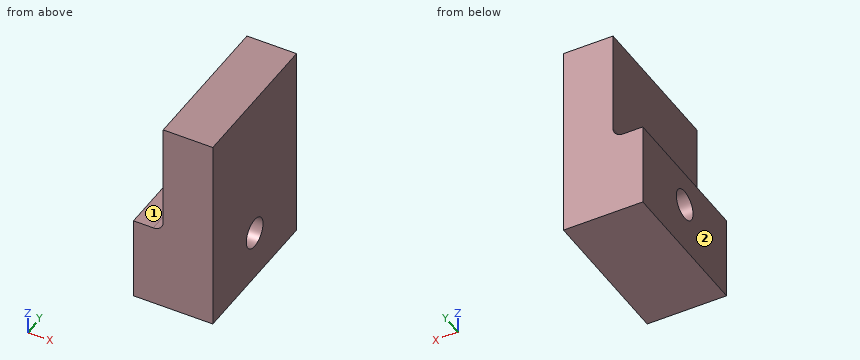
```python
from build123d import *

# Parameters (mm, degrees)
EXTRUDE_1_DEPTH     = 15
CUT_EXTRUDE_1_DEPTH = 15
FILLET_1_R          = 1


with BuildPart() as part:
    # 草图1 → 凸台-拉伸1 (new body)
    with BuildSketch(Plane(origin=(0, 0, 0), x_dir=(1, 0, 0), z_dir=(0, 1, 0))):
        Polygon((-5.74789916, 13.058823529), (2.25210084, 13.058823529), (2.25210084, -6.941176471), (-2.74789916, -6.941176471), (-2.74789916, 4.558823529), (-5.74789916, 4.558823529), align=None)
    extrude(amount=EXTRUDE_1_DEPTH)

    # 草图2 → 切除-拉伸1 (cut)
    with BuildSketch(Plane.ZY.offset(5.74789916)):
        with BuildLine():
            ThreePointArc((-6.558823529, 7.5), (-8.058823529, 9), (-9.558823529, 7.5))
            Line((-9.558823529, 7.5), (-6.558823529, 7.5))
        make_face()
        with BuildLine():
            Line((-6.558823529, 7.5), (-9.558823529, 7.5))
            ThreePointArc((-9.558823529, 7.5), (-8.058823529, 6), (-6.558823529, 7.5))
        make_face()
    extrude(amount=-CUT_EXTRUDE_1_DEPTH, mode=Mode.SUBTRACT)

    # 圆角1
    fillet_1_edges = [part.edges().sort_by_distance(p)[0] for p in [
        (-2.74789916, 7.5, -4.558823529),
    ]]
    fillet(fillet_1_edges, radius=FILLET_1_R)


solid = part.part
```
Geometry check sheet. Reference: the model listing, model coordinates, mm. Face numbers are marked on the shaded views. A direction names the side the tool comes from. Coordinates: 2 decimals unless noted, no trailing zeros. Write each loop counter-clockwise with the first axis right and the second up, starting at its lowest first coordinate (ties: lowest second). Pieces come first, ordered by that corner, then holes. Notation, with made-up numbers: M 56,-3.75 L 100,-3.75 A13 ccw 100,9.25 Z; hole C 48,-23.75 d6. An arc over 180 degrees is marked long. Answer as a JSON object with one key per item and string values.
1. Tool access check on the marked faces 1 and 2. Record the directions out of +Z, -Z, +X, -X, +Y, -Y that give a thin tool (end or side, any length) a straight path to the whole face; none if there is none.
Answers below:
{"face 1": "+Z, -X, +Y, -Y", "face 2": "+Z, -Z, -X, +Y, -Y"}
2. Section check D-D, the plane z = 0. Enter the section's corners in (x, y).
Answers below:
{"outline": "M -2.75,0 L 2.25,0 L 2.25,15 L -2.75,15 Z"}
3. Section check C-C, the plane y = 9.5. Enter the section's corners in (x, z), plus the area to 3 significant figures.
Answers below:
{"outline": "M -5.75,-13.06 L 2.25,-13.06 L 2.25,6.94 L -2.75,6.94 L -2.75,-3.56 A1 cw -3.75,-4.56 L -5.75,-4.56 Z", "area": "126 mm²"}
4. Scan lines: L1, parallel to Z at x = 0.5, y = 7.5; L2, parallel to X at y = 13, z = 4.75; L3, parallel to Z at x = -5, y = 4.5. Record each from-to range of solid material in increasing order.
Answers below:
{"L1": "z = -13.06 to -9.56, -6.56 to 6.94", "L2": "x = -2.75 to 2.25", "L3": "z = -13.06 to -4.56"}
5. Section check B-B, the plane x = -2.25. Enter the section's corners in (y, z), plus the area to 3 significant figures.
Answers below:
{"outline": "M 0,-13.06 L 15,-13.06 L 15,6.94 L 0,6.94 Z; hole C 7.5,-8.06 d3", "area": "293 mm²"}
6. Go/stop test with flat-tipped pins: pin 1 Ø8 at (y, z) = (6.5, -2) entering from -X; pin 2 Ø2 at (x, y) = (-4.5, 7) entering from +Z; pin 3 Ø1.5 at (x, y) = (-4, 11) entering from +Z; pin 4 Ø3 at (y, z) = (5, 1) entering from -X. Record where each tip stops, or that it passes through.
Answers below:
{"pin 1": "stops at x = -5.75", "pin 2": "stops at z = -4.53", "pin 3": "stops at z = -4.43", "pin 4": "stops at x = -2.75"}
7. Section check A-A, the plane y = 7.5. Enter the section's corners in (x, z), plus the area to 3 significant figures.
Answers below:
{"outline": "M -5.75,-13.06 L 2.25,-13.06 L 2.25,-9.56 L -5.75,-9.56 Z; M -5.75,-6.56 L 2.25,-6.56 L 2.25,6.94 L -2.75,6.94 L -2.75,-3.56 A1 cw -3.75,-4.56 L -5.75,-4.56 Z", "area": "102 mm²"}
